```python
from build123d import *

# Parameters (mm, degrees)
EXTRUDE_1_DEPTH     = 20
SKETCH_3_R          = 2.45
CUT_EXTRUDE_1_DEPTH = 2.999162
SKETCH_5_R          = 2.45
CUT_EXTRUDE_2_DEPTH = 2.994438
FILLET_1_R          = 2
FILLET_2_R          = 2


with BuildPart() as part:
    # 草图1 → 凸台-拉伸1 (new body)
    with BuildSketch(Plane.XY):
        Polygon((0, 0), (20.001593334, 0), (20.001593334, 2.994438252), (2.999161685, 2.994438252), (2.999161685, 19.996869901), (0, 19.996869901), align=None)
    extrude(amount=EXTRUDE_1_DEPTH)

    # 草图3 → 切除-拉伸1 (cut)
    with BuildSketch(Plane(origin=(2.999161685, 0, 0), x_dir=(0, 0, -1), z_dir=(1, 0, 0))):
        with Locations((-10, 9.996869901)):
            Circle(SKETCH_3_R)
    extrude(amount=-CUT_EXTRUDE_1_DEPTH, mode=Mode.SUBTRACT)

    # 草图5 → 切除-拉伸2 (cut)
    with BuildSketch(Plane(origin=(0, 2.994438252, 0), x_dir=(1, 0, 0), z_dir=(0, 1, 0))):
        with Locations((10.001593334, -10)):
            Circle(SKETCH_5_R)
    extrude(amount=-CUT_EXTRUDE_2_DEPTH, mode=Mode.SUBTRACT)

    # 圆角1
    fillet_1_edges = [part.edges().sort_by_distance(p)[0] for p in [
        (2.999161685, 19.996869901, 10),
    ]]
    fillet(fillet_1_edges, radius=FILLET_1_R)

    # 圆角2
    fillet_2_edges = [part.edges().sort_by_distance(p)[0] for p in [
        (20.001593334, 2.994438252, 10),
    ]]
    fillet(fillet_2_edges, radius=FILLET_2_R)


solid = part.part
```
The listing builds one solid part. Answer for the finished solid, in the listing's coordinates (mm). A direction names the side the tool comes from. Round coordinates to 2 decimals unless told otherwise and drop trailing zeros. Order: outer loops, then holes, each group sorted by start corner. A loop starts at its lowest first (then second) coordinate and runs counter-clockwise, first axis right, second up. Notation, with made-up numbers: (5.25, 32.5) -> (61.25, 32.5) arc R20 ccw to (61.25, 43.5) -> close; hole circle Ø2 at (-39.5, 18). An arc over 180 degrees is marked (long way). Answer as CSV lines item,"result".
Q1. A cutting plane is placed at B-B on y = 11.5. Determine the outline of the cut face in (x, z).
Computed values:
outline,"(0, 0) -> (3, 0) -> (3, 8.07) -> (0, 8.07) -> close; (0, 11.93) -> (3, 11.93) -> (3, 20) -> (0, 20) -> close"
Q2. A cutting plane is placed at A-A on z = 10. Determine the outline of the cut face in (x, y), plus the area to 3 significant figures.
Computed values:
outline,"(0, 0) -> (7.55, 0) -> (7.55, 2.99) -> (3, 2.99) -> (3, 7.55) -> (0, 7.55) -> close; (0, 12.45) -> (3, 12.45) -> (3, 18) arc R2 ccw to (1, 20) -> (0, 20) -> close; (12.45, 0) -> (20, 0) -> (20, 0.99) arc R2 ccw to (18, 2.99) -> (12.45, 2.99) -> close"
area,"79.8 mm^2"
Q3. Which of the six approach directions +Z, -Z, +X, -X, +Y, -Y give full straight-line access (tool end or side, diameter ignored) to faces 1 (the flat face through (2.5, 5.6, 0)), 2 (the flat face through (2.999, 12, 8))?
Computed values:
face 1,"-Z, +X, -X, +Y, -Y"
face 2,"+Z, -Z, +X, +Y"
Q4. For a pull along Z with two mould halves and no side action, classify faces 3 (the cylindrical face through (1.52, 11.65, 11.81)), 4 (the flat face through (2.5, 5.6, 20)), 5 (the cylindrical face through (9.5, 1.5, 12.4)), 6 (the cylindrical face through (19.4, 2.424, 10.14)) as +Z half, -Z half, draft (parallel to the pull), parting line (faces both ways), or undercut.
Computed values:
face 3,"undercut"
face 4,"+Z half"
face 5,"undercut"
face 6,"draft"
Q5. A cutting plane is placed at C-C on x = 8. Determine the outline of the cut face in (y, z), plus the area to 3 significant figures.
Computed values:
outline,"(0, 0) -> (2.99, 0) -> (2.99, 8.59) -> (0, 8.59) -> close; (0, 11.41) -> (2.99, 11.41) -> (2.99, 20) -> (0, 20) -> close"
area,"51.4 mm^2"
Q6. Given pin 1 (10 mm diameter, centred on y = 6, z = 10, fed in from +X); pin 2 (7.5 mm diameter, centred on x = 12, z = 13, fed in from +Y); pin 3 (5 mm diameter, centred on y = 8, z = 10.5, fed in from +X); pin 4 (4 mm diameter, centred on y = 10, z = 10, fed in from -X), each flat-ended and moving along its own axis, determine where each tip first touches the part or whether it passes through.
Computed values:
pin 1,"stops at x = 20"
pin 2,"stops at y = 2.99"
pin 3,"stops at x = 3"
pin 4,"passes through"
Q7. A cutting plane is placed at D-D on z = 17. Determine the outline of the cut face in (x, y), plus the area to 3 significant figures.
Computed values:
outline,"(0, 0) -> (20, 0) -> (20, 0.99) arc R2 ccw to (18, 2.99) -> (3, 2.99) -> (3, 18) arc R2 ccw to (1, 20) -> (0, 20) -> close"
area,"109 mm^2"
Q8. Consider line 1 (Y direction, x = 0.65, z = 10); line 2 (Y direction, x = 4.25, z = 15). Determine where each line is inside the solid, lowest interval first. Write a range as from..to.
Computed values:
line 1,"y = 0..7.55, 12.45..20"
line 2,"y = 0..2.99"
